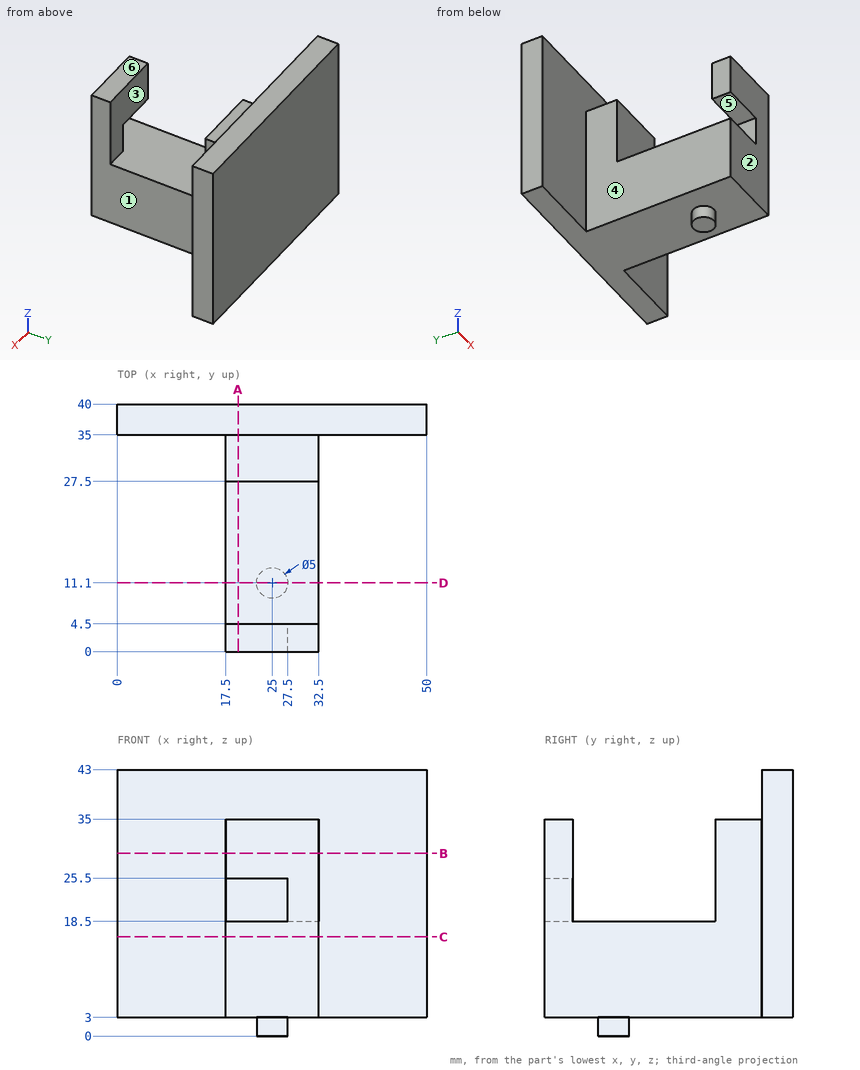
The drawing under review shows one solid part. Ordinate dimensions are in mm from its lowest x, y, z. A direction names the side the tool comes from. Round coordinates to 2 decimals unless told otherwise and drop trailing zeros. Order: outer loops, then holes, each group sorted by start corner. A loop starts at its lowest first (then second) coordinate and runs counter-clockwise, first axis right, second up. Notation, with made-up numbers: M 60,71.25 L 67,71.25 A24 ccw 67,102.25 Z; hole C -4,60 d1. An arc over 180 degrees is marked long. Answer as CSV lines item,"result". Start each with the question number.
1) Tool access review of the marked faces 4, 5 and 6: name each direction out of +Z, -Z, +X, -X, +Y, -Y from which nothing blocks a thin tool from reaching the whole face with its end or side.
2) The part is to be moulded in two halves that separate along Y. For the marked faces 1, 2 and 3, say which applies: +Y half, -Y half, draft (parallel to the pull), parting line (faces both ways), or undercut.
3) Add section C-C (z = 16). Give the boundary of the cut face in (x, y), then the cut area to 3 significant figures.
4) For pin 1 Ø1.3 at (y, z) = (1.5, 29) entering from -X; pin 2 Ø6 at (x, y) = (23.5, 32.5) entering from +Z; pin 3 Ø12 at (x, y) = (27, 17) entering from +Z; pin 4 Ø5 at (x, y) = (22.5, 3.5) entering from -Z, all flat-tipped, find the tip position at first contact; note any pin that passes through.
5) Add section A-A (x = 19.5). Give the boundary of the cut face in (y, z).
6) Add section D-D (y = 11.1). Give the boundary of the cut face in (x, z), then the cut area to 4 significant figures.
7) Wall thickness on line 1 along Y through (x, z) = (44.5, 21.5); line 2 along Z through (x, y) = (25, 5.5); line 3 along Y through (x, z) = (21.5, 27): over which ranges is each line inside the solid? List them lowest first. Write a range as [from, to].
8) Add section B-B (z = 29.5). Give the boundary of the cut face in (x, y), then the cut area to 3 significant figures.
Resolved:
1,face 4,"+Z, -Z, -X, -Y"
1,face 5,"-X, -Y"
1,face 6,"+Z, +X, -X, -Y"
2,face 1,"draft"
2,face 2,"-Y half"
2,face 3,"undercut"
3,outline,"M 0,35 L 17.5,35 L 17.5,0 L 32.5,0 L 32.5,35 L 50,35 L 50,40 L 0,40 Z"
3,area,"775 mm^2"
4,pin 1,"x = 17.5"
4,pin 2,"z = 43"
4,pin 3,"z = 18.5"
4,pin 4,"z = 3"
5,outline,"M 0,3 L 40,3 L 40,43 L 35,43 L 35,35 L 27.5,35 L 27.5,18.5 L 0,18.5 Z; M 0,25.5 L 4.5,25.5 L 4.5,35 L 0,35 Z"
6,outline,"M 17.5,3 L 22.5,3 L 22.5,0 L 27.5,0 L 27.5,3 L 32.5,3 L 32.5,18.5 L 17.5,18.5 Z"
6,area,"247.5 mm^2"
7,line 1,"[35, 40]"
7,line 2,"[3, 18.5]"
7,line 3,"[0, 4.5], [27.5, 40]"
8,outline,"M 0,35 L 17.5,35 L 17.5,27.5 L 32.5,27.5 L 32.5,35 L 50,35 L 50,40 L 0,40 Z; M 17.5,0 L 32.5,0 L 32.5,4.5 L 17.5,4.5 Z"
8,area,"430 mm^2"
